Read the model definition and answer for the solid it produces. Units are mm, in the model's axes. A direction names the side the tool comes from. Coordinates: 2 decimals unless noted, no trailing zeros. Order: outer loops, then holes, each group sorted by start corner. A loop starts at its lowest first (then second) coordinate and runs counter-clockwise, first axis right, second up. Notation, with made-up numbers: (-13.5, -10) -> (42.5, -10) arc R18 cw to (42.5, 18) -> close; hole circle Ø5 at (38, -17). An arc over 180 degrees is marked (long way). Answer in a Markdown table with one row per item.
from build123d import *

# Parameters (mm, degrees)
F0_W      = 26
F0_H      = 26
F0_W_2    = 16
F0_H_2    = 16
F1_DEPTH  = 2
F2_DEPTH  = 20
F3_W      = 26
F3_H      = 26
F3_W_2    = 18
F3_H_2    = 18
F4_DEPTH  = 4
F5_W      = 5
F5_H      = 4
F6_DEPTH  = 4
F7_D      = 2.7
F7_DEPTH  = 4
F7_TIP    = 0.8111618357
F9_W      = 8
F9_H      = 6
F10_DEPTH = 10.28
F9_W_2    = 16
F9_H_2    = 10
F11_DEPTH = 120


with BuildPart() as f1:
    # F0 (on Top) → F1 (new body)
    with BuildSketch(Plane.XY):
        Rectangle(F0_W, F0_H)
        Rectangle(F0_W_2, F0_H_2, mode=Mode.SUBTRACT)
        Rectangle(F0_W_2, F0_H_2)
    extrude(amount=F1_DEPTH)

    # F0 (on Top) → F2 (join)
    with BuildSketch(Plane.XY):
        Rectangle(F0_W, F0_H)
        Rectangle(F0_W_2, F0_H_2, mode=Mode.SUBTRACT)
    extrude(amount=F2_DEPTH)

    # F3 (on face) → F4 (join)
    with BuildSketch(Plane.XY.offset(20)):
        Rectangle(F3_W, F3_H)
        Rectangle(F3_W_2, F3_H_2, mode=Mode.SUBTRACT)
    extrude(amount=F4_DEPTH)

    # F5 (on face) → F6 (cut, through all)
    with BuildSketch(Plane.XY.offset(24)):
        with Locations((0, -11)):
            Rectangle(F5_W, F5_H)
        with Locations((0, 11)):
            Rectangle(F5_W, F5_H)
    extrude(amount=-F6_DEPTH, mode=Mode.SUBTRACT)

    # F7
    with Locations(Plane.XY.offset(24)):
        with Locations((-10.5, 10.5), (10.5, 10.5), (-10.5, -10.5), (10.5, -10.5)):
            Hole(F7_D / 2, depth=F7_DEPTH)
            with Locations((0, 0, -(F7_DEPTH + F7_TIP / 2))):  # 118° drill point
                Cone(0, F7_D / 2, F7_TIP, mode=Mode.SUBTRACT)

    # F9 (on face) → F10 (cut)
    with BuildSketch(Plane(origin=(0, 13, 0), x_dir=(-1, 0, 0), z_dir=(0, 1, 0))):
        with Locations((0, 5)):
            Rectangle(F9_W, F9_H)
    extrude(amount=-F10_DEPTH, mode=Mode.SUBTRACT)

    # F9 (on face) → F11 (join)
    with BuildSketch(Plane(origin=(0, 13, 0), x_dir=(-1, 0, 0), z_dir=(0, 1, 0))):
        with Locations((0, 5)):
            Rectangle(F9_W_2, F9_H_2)
        with Locations((0, 5)):
            Rectangle(F9_W, F9_H, mode=Mode.SUBTRACT)
    extrude(amount=F11_DEPTH)


solid = f1.part
Q1. For faces 5 (the face through (8, 72, 5)), 6 (the face through (8, 0, 11)), 7 (the face through (4, 70, 5)), 8 (the face through (0, -13, 12)), determine the directions among +Z, -Z, +X, -X, +Y, -Y from which every point of the face is accessible in a straight line to the end or side of a thin tool.
Outcome:
| item | result |
|---|---|
| face 5 | +Z, -Z, +X, +Y |
| face 6 | +Z |
| face 7 | +Y |
| face 8 | +Z, -Z, +X, -X, -Y |
Q2. The part is cut by section A-A (x = -0.75). Write down the section's boundary in (y, z).
Outcome:
| item | result |
|---|---|
| outline | (-13, 0) -> (133, 0) -> (133, 2) -> (-8, 2) -> (-8, 20) -> (-13, 20) -> close; (8, 8) -> (133, 8) -> (133, 10) -> (13, 10) -> (13, 20) -> (8, 20) -> close |
Q3. Given pin 1 (11 mm diameter, centred on y = 77, z = 3.5, fed in from +X); pin 2 (1.2 mm diameter, centred on x = -5.5, z = 23, fed in from +Y); pin 3 (2 mm diameter, centred on x = 10.5, y = -10.5, fed in from +Z), each flat-ended and moving along its own axis, determine where each tip first touches the part or whether it passes through.
Outcome:
| item | result |
|---|---|
| pin 1 | x = 8 |
| pin 2 | y = 13 |
| pin 3 | z = 19.79 |
Q4. The part is cut by section D-D (y = 2). Write down the section's boundary in (x, z).
Outcome:
| item | result |
|---|---|
| outline | (-13, 0) -> (13, 0) -> (13, 24) -> (9, 24) -> (9, 20) -> (8, 20) -> (8, 2) -> (-8, 2) -> (-8, 20) -> (-9, 20) -> (-9, 24) -> (-13, 24) -> close |
Q5. For a pull along X with two mould halves and no side action, classify faces 1 (the face through (10.72, 10.41, 19.33)), 2 (the face through (-11.226, 11.638, 21.972)), 3 (the face through (0.1, 133, 8.4)), 4 (the face through (-8, 72, 5)) as pulls with the +X half, pulls with the -X half, needs draft (parallel to the pull), parting line crosses it, or undercut.
Outcome:
| item | result |
|---|---|
| face 1 | undercut |
| face 2 | undercut |
| face 3 | needs draft |
| face 4 | pulls with the -X half |
Q6. The part is cut by section B-B (y = 120). Write down the section's boundary in (x, z).
Outcome:
| item | result |
|---|---|
| outline | (-8, 0) -> (8, 0) -> (8, 10) -> (-8, 10) -> close; hole (-4, 2) -> (4, 2) -> (4, 8) -> (-4, 8) -> close |
Q7. Consider line 1 (X direction, y = 10.5, z = 23.15); line 2 (Y direction, x = 10.5, z = 22.55); line 3 (Y direction, x = -0.25, z = 13.5). Determine where each line is inside the solid, lowest interval first.
Outcome:
| item | result |
|---|---|
| line 1 | -13 to -11.85, -9.15 to -2.5, 2.5 to 9.15, 11.85 to 13 |
| line 2 | -13 to -11.85, -9.15 to 9.15, 11.85 to 13 |
| line 3 | -13 to -8, 8 to 13 |
Q8. The part is cut by section C-C (x = 5.5). Write down the section's boundary in (y, z).
Outcome:
| item | result |
|---|---|
| outline | (-13, 0) -> (133, 0) -> (133, 10) -> (13, 10) -> (13, 24) -> (9, 24) -> (9, 20) -> (8, 20) -> (8, 2) -> (-8, 2) -> (-8, 20) -> (-9, 20) -> (-9, 24) -> (-13, 24) -> close |
